Read the model definition and answer for the solid it produces. Units are mm, in the model's axes. A direction names the side the tool comes from. Coordinates: 2 decimals unless noted, no trailing zeros. Order: outer loops, then holes, each group sorted by start corner. A loop starts at its lowest first (then second) coordinate and runs counter-clockwise, first axis right, second up. Notation, with made-up numbers: (1, -2) - (28, -2) arc R23 ccw to (28, 6) - close; hole circle Ø4 at (56.5, 1). An arc over 180 degrees is marked (long way). Write item = value, one per line.
from build123d import *

# Parameters (mm, degrees)
SKETCH_W        = 40
SKETCH_H        = 60
PAD_DEPTH       = 5
SKETCH001_W     = 10
SKETCH001_H     = 40
POCKET_DEPTH    = 2
SKETCH002_R     = 4
POCKET001_DEPTH = 2
SKETCH003_W     = 15
SKETCH003_H     = 5
POCKET002_DEPTH = 2
SKETCH004_R     = 2.5
POCKET003_DEPTH = 5
SKETCH005_W     = 4
SKETCH005_H     = 4
POCKET004_DEPTH = 2
SKETCH006_R     = 2.5
POCKET005_DEPTH = 3
FILLET_R        = 2
FILLET001_R     = 0.5
SKETCH012_R     = 2.5
POCKET008_DEPTH = 5
FILLET005_R     = 5


with BuildPart() as part:
    # Sketch → Pad (new body)
    with BuildSketch(Plane.XY):
        Rectangle(SKETCH_W, SKETCH_H)
    extrude(amount=PAD_DEPTH)

    # Sketch001 (on Face6 of Pad) → Pocket (cut)
    with BuildSketch(Plane.XY.offset(5)):
        Rectangle(SKETCH001_W, SKETCH001_H)
    extrude(amount=-POCKET_DEPTH, mode=Mode.SUBTRACT)

    # Sketch002 (on Face5 of Pocket) → Pocket001 (cut)
    with BuildSketch(Plane.XY.offset(5)):
        with Locations((9, 0)):
            Circle(SKETCH002_R)
        with Locations((-9, 0)):
            Circle(SKETCH002_R)
    extrude(amount=-POCKET001_DEPTH, mode=Mode.SUBTRACT)

    # Sketch003 (on Face5 of Pocket001) → Pocket002 (cut)
    with BuildSketch(Plane.XY.offset(5)):
        Rectangle(SKETCH003_W, SKETCH003_H)
    extrude(amount=-POCKET002_DEPTH, mode=Mode.SUBTRACT)

    # Sketch004 (on Face22 of Pocket002) → Pocket003 (cut)
    with BuildSketch(Plane.XY.offset(3)):
        with Locations((0, -12)):
            Circle(SKETCH004_R)
    extrude(amount=-POCKET003_DEPTH, mode=Mode.SUBTRACT)

    # Sketch005 (on Face5 of Pocket003) → Pocket004 (cut)
    with BuildSketch(Plane.XY.offset(5)):
        with Locations((0, -20)):
            Rectangle(SKETCH005_W, SKETCH005_H)
    extrude(amount=-POCKET004_DEPTH, mode=Mode.SUBTRACT)

    # Sketch006 (on Face31 of Pocket004) → Pocket005 (cut)
    with BuildSketch(Plane.XY.offset(3)):
        with Locations((0, 14)):
            Circle(SKETCH006_R)
    extrude(amount=-POCKET005_DEPTH, mode=Mode.SUBTRACT)

    # Fillet
    fillet_edges = [part.edges().sort_by_distance(p)[0] for p in [
        (-5, 20, 4),
        (5, 20, 4),
        (-5, -20, 4),
        (5, -20, 4),
    ]]
    fillet(fillet_edges, radius=FILLET_R)

    # Fillet001
    fillet001_edges = [part.edges().sort_by_distance(p)[0] for p in [
        (-2, -22, 4),
        (2, -22, 4),
        (2, -20, 4),
        (-2, -20, 4),
    ]]
    fillet(fillet001_edges, radius=FILLET001_R)

    # Sketch012 (on Face1 of Fillet001) → Pocket008 (cut)
    with BuildSketch(Plane.XY.offset(5)):
        with Locations((-12, 22)):
            Circle(SKETCH012_R)
        with Locations((12, 22)):
            Circle(SKETCH012_R)
    pocket008 = extrude(amount=-POCKET008_DEPTH, mode=Mode.SUBTRACT)

    # Mirrored: Pocket008 across XZ
    add(pocket008.mirror(Plane.XZ), mode=Mode.SUBTRACT)

    # Fillet005
    fillet005_edges = [part.edges().sort_by_distance(p)[0] for p in [
        (-20, -30, 2.5),
        (20, -30, 2.5),
        (-20, 30, 2.5),
        (20, 30, 2.5),
    ]]
    fillet(fillet005_edges, radius=FILLET005_R)


solid = part.part
1) Determine the mould class of faces 1 (the face through (4.4, -19.43, 3.99)), 2 (the face through (-20, 0, 2)), 3 (the face through (-19, 28, 3)) for opening direction Y: pulls with the +Y half, pulls with the -Y half, needs draft (parallel to the pull), parting line crosses it, or undercut.
Returned:
face_1 = undercut
face_2 = needs draft
face_3 = pulls with the +Y half
2) The part is cut by section C-C (z = 0.75). Determine the outline of the cut face in (x, y).
Returned:
outline = (-20, -25) arc R5 ccw to (-15, -30) - (15, -30) arc R5 ccw to (20, -25) - (20, 25) arc R5 ccw to (15, 30) - (-15, 30) arc R5 ccw to (-20, 25) - close; hole circle Ø5 at (-12, -22); hole circle Ø5 at (-12, 22); hole circle Ø5 at (0, -12); hole circle Ø5 at (0, 14); hole circle Ø5 at (12, -22); hole circle Ø5 at (12, 22)
3) Straight lines are drawn through the part: line 1 along Y through (x, z) = (0, 2.1); line 2 along X through (y, z) = (-22, 1.3); line 3 along Y through (x, z) = (12, 2.3). For each, find the intervals that lie inside material, in ascending order. Write a range as from..to.
Returned:
line_1 = -30..-14.5, -9.5..11.5, 16.5..30
line_2 = -20..-14.5, -9.5..9.5, 14.5..20
line_3 = -30..-24.5, -19.5..19.5, 24.5..30
4) The part is cut by section D-D (y = 5.5). Determine the outline of the cut face in (x, z).
Returned:
outline = (-20, 0) - (20, 0) - (20, 5) - (5, 5) - (5, 3) - (-5, 3) - (-5, 5) - (-20, 5) - close
5) For faces 4 (the face through (-4.43, -19.4, 3.99)), 5 (the face through (20, 0, 2)), determine the directions among +Z, -Z, +X, -X, +Y, -Y from which every point of the face is accessible in a straight line to the end or side of a thin tool.
Returned:
face_4 = +Z
face_5 = +Z, -Z, +X, +Y, -Y
6) The part is cut by section A-A (x = 0). Determine the outline of the cut face in (y, z).
Returned:
outline = (-30, 0) - (-14.5, 0) - (-14.5, 3) - (-22, 3) - (-22, 5) - (-30, 5) - close; (-9.5, 0) - (11.5, 0) - (11.5, 3) - (-9.5, 3) - close; (16.5, 0) - (30, 0) - (30, 5) - (20, 5) - (20, 3) - (16.5, 3) - close
7) The part is cut by section B-B (y = 22). Determine the outline of the cut face in (x, z), and give its area (3 significant figures).
Returned:
outline = (-20, 0) - (-14.5, 0) - (-14.5, 5) - (-20, 5) - close; (-9.5, 0) - (9.5, 0) - (9.5, 5) - (-9.5, 5) - close; (14.5, 0) - (20, 0) - (20, 5) - (14.5, 5) - close
area = 150 mm^2
8) Flat-ended cylindrical pins translate along their axes: pin 1 Ø4.5 at (x, y) = (0, 14) entering from +Z; pin 2 Ø8 at (x, y) = (0, -12) entering from +Z. Find the tip coordinate at first contact, or state that the pin passes through.
Returned:
pin_1 = through
pin_2 = 3
